Verification items for the finished model (mm, model axes). Round coordinates to 2 decimals unless told otherwise and drop trailing zeros. Write each loop counter-clockwise with the first axis right and the second up, starting at its lowest first coordinate (ties: lowest second). Pieces come first, ordered by that corner, then holes. Notation, with made-up numbers: (-16.75, -15.75) - (21.25, -15.75) arc R27 ccw to (21.25, 1.25) - close; hole circle Ø6 at (16.25, 25.25). An arc over 180 degrees is marked (long way). Answer as a JSON object with one key per item and string values. Group by question number.
1) Go/stop test with a flat-tipped pin: pin 1 Ø1.5 at (y, z) = (30.5, -1) entering from -X. Record where the tip stops, or that it passes through.
2) Thickness scan on line 1 (X direction, y = 90, z = -0.15); line 2 (X direction, y = 25.5, z = 1.9); line 3 (Z direction, x = 0.5, y = -97). Record the ranges inside material, lowest first.
3) Section check C-C (x = -11.5). Enter the section's corners in (y, z) (3 decimals), then the cut area to 3 significant figures.
4) Section check B-B (y = -59). Enter the section's corners in (x, z).
5) Section check A-A (z = 0). Enter the section's corners in (x, y), then the cut area to 3 significant figures.
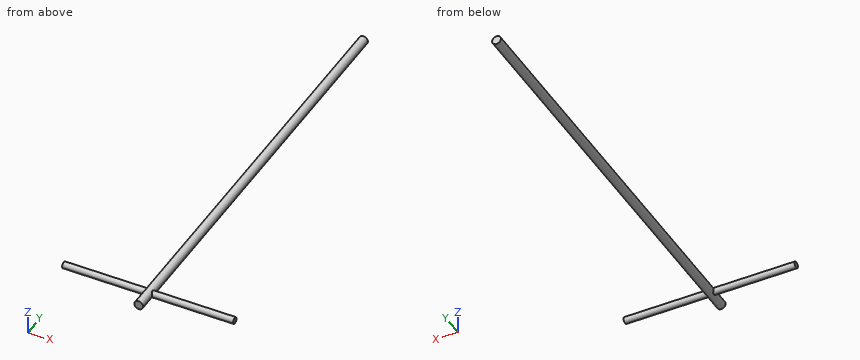
```python
from build123d import *

# Parameters (mm, degrees)
F1_DEPTH      = 127
F1_DEPTH_BACK = 127
F4_DEPTH      = 50.8
F4_DEPTH_BACK = 50.8


with BuildPart() as f1:
    # F0 (on Front) → F1 (new body, two sides)
    with BuildSketch(Plane.XZ) as f1_sk:
        with BuildLine():
            Line((0, -2.6035), (0, 2.6035))
            ThreePointArc((0, 2.6035), (-2.6035, 0), (0, -2.6035))
        make_face()
    extrude(amount=F1_DEPTH)
    extrude(f1_sk.sketch, amount=-F1_DEPTH_BACK)

    # F3: F1 across plane


with BuildPart() as f1_1:
    add(f1.part)
    add(f1.part.mirror(Plane.YZ))

    # F2 (on face) → F4 (join, two sides)
    with BuildSketch(Plane.YZ) as f4_sk:
        with BuildLine():
            Line((-116.9321797776, 0), (-113.1221797776, 0))
            ThreePointArc((-113.1221797776, 0), (-115.0271797776, 1.905), (-116.9321797776, 0))
        make_face()
        with BuildLine():
            ThreePointArc((-116.9321797776, 0), (-115.0271797776, -1.905), (-113.1221797776, 0))
            Line((-113.1221797776, 0), (-116.9321797776, 0))
        make_face()
    extrude(amount=F4_DEPTH)
    extrude(f4_sk.sketch, amount=-F4_DEPTH_BACK)


solid = f1_1.part
```
Returned:
{
 "1": {"pin 1": "x = -2.59"},
 "2": {"line 1": "-2.6 to 2.6", "line 2": "-1.78 to 1.78", "line 3": "-2.56 to 2.56"},
 "3": {"outline": "circle Ø3.81 at (-115.027, 0)", "area": "11.4 mm2"},
 "4": {"outline": "circle Ø5.21 at (0, 0)"},
 "5": {"outline": "(-50.8, -116.93) - (-2.6, -116.93) - (-2.6, -127) - (2.6, -127) - (2.6, -116.93) - (50.8, -116.93) - (50.8, -113.12) - (2.6, -113.12) - (2.6, 127) - (-2.6, 127) - (-2.6, -113.12) - (-50.8, -113.12) - close", "area": "1,690 mm2"}
}
